from build123d import *

# Parameters (mm, degrees)
SKETCH1_W            = 14.8
SKETCH1_H            = 17.7
SKETCH1_R            = 1.65
BOSS_EXTRUDE1_DEPTH  = 2.5
FILLET1_R            = 1
SKETCH6_W            = 16.5
SKETCH6_H            = 20
BOSS_EXTRUDE8_DEPTH  = 2.5
SKETCH7_W            = 13.5
SKETCH7_H            = 20
SKETCH7_W_2          = 2.5
BOSS_EXTRUDE9_DEPTH  = 3.5
FILLET5_R            = 2
FILLET6_R            = 1
SKETCH10_W           = 14.5
SKETCH10_H           = 15.3
BOSS_EXTRUDE10_DEPTH = 2.5
SKETCH11_W           = 5.5
SKETCH11_H           = 15.3
BOSS_EXTRUDE11_DEPTH = 1.5
FILLET7_R            = 1
FILLET8_R            = 4


with BuildPart() as part:
    # Sketch1 → Boss-Extrude1 (new body)
    # profile 1 of 2: a face of its own
    with BuildSketch(Plane.XY):
        with Locations((-5.7, 7.65)):
            Rectangle(SKETCH1_W, SKETCH1_H)
    # profile 2 of 2: a face of its own
    with BuildSketch(Plane.XY):
        Polygon((1.7, -1.2), (-13.1, -1.2), (-13.1, -16.5), (13.1, -16.5), (13.1, -1.2), align=None)
        with Locations((-8.1, -8.5)):
            Circle(SKETCH1_R, mode=Mode.SUBTRACT)
        with Locations((8.1, -8.5)):
            Circle(SKETCH1_R, mode=Mode.SUBTRACT)
    extrude(amount=BOSS_EXTRUDE1_DEPTH)

    # Fillet1
    fillet1_edges = [part.edges().sort_by_distance(p)[0] for p in [
        (1.7, 16.5, 1.25),
        (-13.1, 16.5, 1.25),
    ]]
    fillet(fillet1_edges, radius=FILLET1_R)

    # Sketch6 → Boss-Extrude8 (add)
    with BuildSketch(Plane.ZY.offset(13.1)):
        with Locations((-5.75, -6.5)):
            Rectangle(SKETCH6_W, SKETCH6_H)
    extrude(amount=BOSS_EXTRUDE8_DEPTH)

    # Sketch7 → Boss-Extrude9 (add)
    # profile 1 of 2: a face of its own
    with BuildSketch(Plane(origin=(0, 0, -14), x_dir=(-1, 0, 0), z_dir=(0, 0, -1))):
        with Locations((22.35, -6.5)):
            Rectangle(SKETCH7_W, SKETCH7_H)
        with BuildLine():
            ThreePointArc((20.2, -5.1), (22.9, -2.4), (25.6, -5.1))
            Line((25.6, -5.1), (25.6, -10.5))
            ThreePointArc((25.6, -10.5), (22.9, -13.2), (20.2, -10.5))
            Line((20.2, -10.5), (20.2, -5.1))
        make_face(mode=Mode.SUBTRACT)
    # profile 2 of 2: a face of its own
    with BuildSketch(Plane(origin=(0, 0, -14), x_dir=(-1, 0, 0), z_dir=(0, 0, -1))):
        with Locations((14.35, -6.5)):
            Rectangle(SKETCH7_W_2, SKETCH7_H)
    extrude(amount=BOSS_EXTRUDE9_DEPTH)

    # Fillet5
    fillet5_edges = [part.edges().sort_by_distance(p)[0] for p in [
        (-13.1, -6.5, 0),
        (-15.6, -6.5, -14),
    ]]
    fillet(fillet5_edges, radius=FILLET5_R)

    # Fillet6
    fillet6_edges = [part.edges().sort_by_distance(p)[0] for p in [
        (-13.1, 3.5, 1.25),
        (-15.6, -6.5, 2.5),
    ]]
    fillet(fillet6_edges, radius=FILLET6_R)

    # Sketch10 → Boss-Extrude10 (add)
    with BuildSketch(Plane(origin=(13.1, 0, 0), x_dir=(0, 0, -1), z_dir=(1, 0, 0))):
        with Locations((4.75, -8.85)):
            Rectangle(SKETCH10_W, SKETCH10_H)
    extrude(amount=BOSS_EXTRUDE10_DEPTH)

    # Sketch11 → Boss-Extrude11 (add)
    with BuildSketch(Plane(origin=(0, 0, -12), x_dir=(-1, 0, 0), z_dir=(0, 0, -1))):
        with Locations((-14.35, -8.85)):
            Rectangle(SKETCH11_W, SKETCH11_H)
    extrude(amount=-BOSS_EXTRUDE11_DEPTH)

    # Fillet7
    fillet7_edges = [part.edges().sort_by_distance(p)[0] for p in [
        (13.1, -8.85, 0),
        (15.6, -8.85, 2.5),
        (15.6, -8.85, -10.5),
        (13.1, -8.85, -10.5),
        (1.7, -1.2, 1.25),
        (-13.1, -6.5, -17.5),
    ]]
    fillet(fillet7_edges, radius=FILLET7_R)

    # Fillet8
    fillet8_edges = [part.edges().sort_by_distance(p)[0] for p in [
        (-29.1, -16.5, -15.75),
        (-29.1, 3.5, -15.75),
    ]]
    fillet(fillet8_edges, radius=FILLET8_R)


solid = part.part
CAD build for the part. Positions are in the model's coordinates, mm. A direction names the side the tool comes from. Round coordinates to 2 decimals unless told otherwise and drop trailing zeros. Order: outer loops, then holes, each group sorted by start corner. A loop starts at its lowest first (then second) coordinate and runs counter-clockwise, first axis right, second up. Notation, with made-up numbers: M -4.75,-18 L 7.25,-18 A25 cw 7.25,3 Z; hole C -19.75,40 d11. An arc over 180 degrees is marked long. Use one line per item in the form item = value.
Q1. Saw through at D-D on y = -3. Give the cut face in (x, z), then the cut area to 3 significant figures.
Recorded:
outline = M -29.1,-17.5 L -24.6,-17.5 L -24.6,-14 L -29.1,-14 Z; M -21.2,-17.5 L -14.1,-17.5 A1 ccw -13.1,-16.5 L -13.1,-2 A2 cw -11.1,0 L 12.1,0 A1 cw 13.1,-1 L 13.1,-9.5 A1 cw 12.1,-10.5 L 11.6,-10.5 L 11.6,-12 L 17.1,-12 L 17.1,-10.5 L 16.6,-10.5 A1 cw 15.6,-9.5 L 15.6,1.5 A1 ccw 14.6,2.5 L -14.6,2.5 A1 ccw -15.6,1.5 L -15.6,-12 A2 cw -17.6,-14 L -21.2,-14 Z
area = 193 mm^2
Q2. Saw through at A-A on z = -6. Give the cut face in (x, y).
Recorded:
outline = M -15.6,-16.5 L -13.1,-16.5 L -13.1,3.5 L -15.6,3.5 Z; M 13.1,-16.5 L 15.6,-16.5 L 15.6,-1.2 L 13.1,-1.2 Z
Q3. Saw through at C-C on y = -8.5. State how many separate pieces and enclosed holes the cut face has, then the cut area to 3 significant figures.
Recorded:
separate_pieces = 4
enclosed_holes = 0
area = 170 mm^2
Q4. Which spindle directions (+Z, -Z, +X, -X, +Y, -Y) get a long thin tool onto all of the face, cutting with end or side? Do faces 4 (the flat face through (15.6, -9, -4)), 5 (the flat face through (-20.2, -8, -16)), 6 (the flat face through (-26, -6, -14)), 7 (the flat face through (11.6, -9, -11)). Say none if no direction does.
Recorded:
face_4 = +Z, +X, +Y, -Y
face_5 = +Z, -Z
face_6 = +Z, -X, +Y, -Y
face_7 = -Z, +Y, -Y
Q5. Probe L1, parallel to Y at x = 8.1, z = 0.7; L2, parallel to Y at x = -8.1, z = 1.3; L3, parallel to Z at x = -18, y = -11. List the from-to ranges inside material, lowest first.
Recorded:
L1 = -16.5 to -10.15, -6.85 to -1.2
L2 = -16.5 to -10.15, -6.85 to 16.5
L3 = -17.5 to -14
Q6. Flat gauge pins, fed straight in: P1, Ø2.5, axis at y = -6, z = -4, coming from the -X side; P2, Ø6, axis at x = -12, y = 11.5, coming from the -Z side; P3, Ø4, axis at y = -9.5, z = -1, coming from the +X side. Where does each tip first touch, or does it go through?
Recorded:
P1 = -15.6
P2 = 0
P3 = 15.6
Q7. Two-plate mould, pull along Y, no slides. Class faces 1 (the flat face through (-29.1, -7, -16)), 2 (the flat face through (14, -1.2, -3)), 3 (the cylindrical face through (7.885, -6.864, 1.232)): +Y half, -Y half, draft (parallel to the pull), parting line (faces both ways), or undercut.
Recorded:
face_1 = draft
face_2 = +Y half
face_3 = undercut
Q8. Saw through at B-B on x = -22.9. Give the cut face in (y, z), then the cut area to 3 significant figures.
Recorded:
outline = M -16.5,-17.5 L -13.2,-17.5 L -13.2,-14 L -16.5,-14 Z; M -2.4,-17.5 L 3.5,-17.5 L 3.5,-14 L -2.4,-14 Z
area = 32.2 mm^2
